Check sheet for the modelled part. Datum: model origin and axes. Units: mm. A direction names the side the tool comes from. Coordinates: 2 decimals unless noted, no trailing zeros. Loops run counter-clockwise (first coordinate to the right, second up) from the corner with the lowest first, then second, coordinate; pieces in that order, holes last. Notation, with made-up numbers: (-40, 65) -> (16, 65) arc R33 ccw to (16, 95) -> close; hole circle Ø4 at (78.25, -2.75). An arc over 180 degrees is marked (long way). Use CSV: the item, a comma, the result in double quotes.
```python
from build123d import *

# Parameters (mm, degrees)
SKETCH1_R           = 11
BOSS_EXTRUDE1_DEPTH = 7
SKETCH2_R           = 4.1
CUT_EXTRUDE1_DEPTH  = 2.5
SKETCH3_R           = 2.15
CUT_EXTRUDE2_DEPTH  = 5.5
FILLET1_R           = 1


with BuildPart() as part:
    # Sketch1 → Boss-Extrude1 (new body)
    with BuildSketch(Plane.XY):
        Circle(SKETCH1_R)
    extrude(amount=BOSS_EXTRUDE1_DEPTH)

    # Sketch2 → Cut-Extrude1 (cut)
    with BuildSketch(Plane.XY.offset(7)):
        Circle(SKETCH2_R)
    extrude(amount=-CUT_EXTRUDE1_DEPTH, mode=Mode.SUBTRACT)

    # Sketch3 → Cut-Extrude2 (cut, through all)
    with BuildSketch(Plane.XY.offset(4.5)):
        Circle(SKETCH3_R)
    extrude(amount=-CUT_EXTRUDE2_DEPTH, mode=Mode.SUBTRACT)

    # Fillet1
    fillet1_edges = [part.edges().sort_by_distance(p)[0] for p in [
        (-4.1, 0, 7),
    ]]
    fillet(fillet1_edges, radius=FILLET1_R)


solid = part.part
```
1) Thickness scan on line 1 along Y through (x, z) = (0, 1.4); line 2 along Y through (x, z) = (0, 5.6); line 3 along X through (y, z) = (1, 3.5). Record the ranges inside material, lowest first. Write a range as from..to.
Answer below:
line 1,"y = -11..-2.15, 2.15..11"
line 2,"y = -11..-4.1, 4.1..11"
line 3,"x = -10.95..-1.9, 1.9..10.95"
2) Draft check along X on faces 1 (the cylindrical face through (-2.38, -10.74, 3.45)), 2 (the flat face through (-0.2, -2.3, 0)), 3 (the cylindrical face through (-0.534, 4.065, 5.26)). Enter one of: released by +X, released by -X, zero draft, split by the parting line, or undercut.
Answer below:
face 1,"split by the parting line"
face 2,"zero draft"
face 3,"undercut"
3) Access from +Z, -Z, +X, -X, +Y, -Y to the whole of each face (thin tool, end or side, straight path). Record for faces 4 (the flat face through (2, -2, 4.5)), 5 (the flat face through (2, -5, 7)).
Answer below:
face 4,"+Z"
face 5,"+Z, +X, -X, +Y, -Y"
4) Go/stop test with flat-tipped pins: pin 1 Ø4 at (x, y) = (-0.5, 0.5) entering from +Z; pin 2 Ø2 at (x, z) = (-7, 5) entering from -Y; pin 3 Ø2 at (x, z) = (-3, 2.5) entering from -Y; pin 4 Ø2.5 at (x, y) = (0, 0) entering from +Z. Record where each tip stops, or that it passes through.
Answer below:
pin 1,"stops at z = 4.5"
pin 2,"stops at y = -9.22"
pin 3,"stops at y = -10.82"
pin 4,"passes through"
5) Cross-section at D-D on x = 6. Record the boundary of the cut face in (y, z), and give its area (3 significant figures).
Answer below:
outline,"(-9.22, 0) -> (9.22, 0) -> (9.22, 7) -> (-9.22, 7) -> close"
area,"129 mm²"
6) Cross-section at C-C on z = 4. Record the boundary of the cut face in (x, y).
Answer below:
outline,"circle Ø22 at (0, 0); hole circle Ø4.3 at (0, 0)"
7) Cross-section at A-A on x = 0. Record the boundary of the cut face in (y, z).
Answer below:
outline,"(-11, 0) -> (-2.15, 0) -> (-2.15, 4.5) -> (-4.1, 4.5) -> (-4.1, 6) arc R1 ccw to (-5.1, 7) -> (-11, 7) -> close; (2.15, 0) -> (11, 0) -> (11, 7) -> (5.1, 7) arc R1 ccw to (4.1, 6) -> (4.1, 4.5) -> (2.15, 4.5) -> close"
